Geometry check sheet. Reference: drawing and pictorial views, mm from the part's lowest x, y, z. A direction names the side the tool comes from. Give positions to 0.01 mm unless a question says otherwise; leave off trailing zeros. Loops run counter-clockwise (first coordinate to the right, second up) from the corner with the lowest first, then second, coordinate; pieces in that order, holes last. Notation, with made-up numbers: (35, 64) -> (82, 64) arc R22 cw to (82, 98) -> close; hole circle Ø3 at (-25.75, 0). An arc over 180 degrees is marked (long way). One line per item, written item: value. Start each with the question number.
(1) Tool access check on the marked faces 1 and 2. Record the directions out of +Z, -Z, +X, -X, +Y, -Y that give a thin tool (end or side, any length) a straight path to the whole face; none if there is none.
(2) Draft check along X on the marked faces 3, 4, 5 and 6. Enter one of: pulls with the +X half, pulls with the -X half, needs draft (parallel to the pull), parting line crosses it, or undercut.
(3) Sectioned sample at A-A, the plane y = 9.75. Record the cut outline in (x, z).
(4) Sectioned sample at C-C, the plane z = 2.15. Record the cut outline in (x, y).
(5) Scan lines: line 1 along X through (y, z) = (8.5, 0.95); line 2 along Y through (x, z) = (11, 1.5); line 3 along Y through (x, z) = (10.5, 2.7). Record each from-to range of solid material in increasing order. Write a range as from..to.
(6) Sectioned sample at B-B, the plane x = 11. Record the cut outline in (y, z).
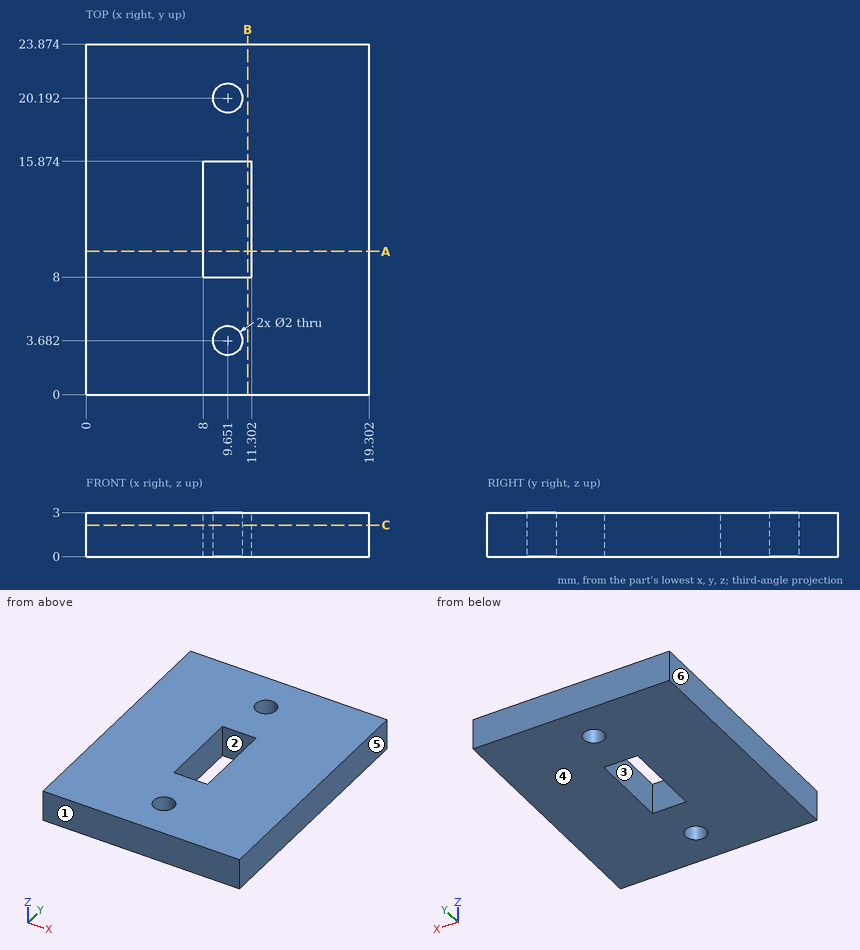
Calculated:
1. face 1: +Z, -Z, +X, -X, -Y
1. face 2: +Z, -Z
2. face 3: undercut
2. face 4: needs draft
2. face 5: pulls with the +X half
2. face 6: pulls with the -X half
3. outline: (0, 0) -> (8, 0) -> (8, 3) -> (0, 3) -> close; (11.3, 0) -> (19.3, 0) -> (19.3, 3) -> (11.3, 3) -> close
4. outline: (0, 0) -> (19.3, 0) -> (19.3, 23.87) -> (0, 23.87) -> close; hole (8, 8) -> (11.3, 8) -> (11.3, 15.87) -> (8, 15.87) -> close; hole circle Ø2 at (9.65, 3.68); hole circle Ø2 at (9.65, 20.19)
5. line 1: x = 0..8, 11.3..19.3
5. line 2: y = 0..8, 15.87..23.87
5. line 3: y = 0..3.15, 4.21..8, 15.87..19.66, 20.72..23.87
6. outline: (0, 0) -> (8, 0) -> (8, 3) -> (0, 3) -> close; (15.87, 0) -> (23.87, 0) -> (23.87, 3) -> (15.87, 3) -> close
